Input: part model. Units: mm. Frame: model coordinates. Face numbers are marked on the shaded views. A direction names the side the tool comes from. Give positions to 0.01 mm unless a question says otherwise; leave off trailing zeros. Loops run counter-clockwise (first coordinate to the right, second up) from the corner with the lowest first, then second, coordinate; pieces in that order, holes last. Notation, with made-up numbers: M 87.5,-30.75 L 101.5,-30.75 A36 ccw 101.5,8.25 Z; hole C 56.5,61 d5. An arc over 180 degrees is marked long. One line per item, written item: value. Start each with the question number.
(1) Access query for the marked faces 1, 2 and 3. Directions: +Z, -Z, +X, -X, +Y, -Y. A direction counts if a zero-diameter tool reaches every point of the face in a straight line with its end or side. Return the directions, or none.
(2) Section B-B on z = -0.05. Output: boundary loops of the cut face in (x, y).
(3) Ray query, line 1 along Y through (x, z) = (0, 0.9); line 2 along Y through (x, z) = (0, -1.2); line 3 along Y through (x, z) = (-15.8, 0.7). Return the intervals inside material, ascending. Write a range as from..to.
(4) Pin query (flat end, axial travel): P1, Ø1.8, axis at x = 1, y = 15, coming from the +Z side; P2, Ø1.5, axis at y = 5.5, z = 1, coming from the -X side; P3, Ø3, axis at x = -15.8, y = 0, coming from the +Z side; P4, Ø1.4, axis at x = -15.5, z = -1, coming from the -Y side. Return the tip coordinate at first contact, or that it passes through.
(5) Section A-A on x = -15.8. Output: boundary loops of the cut face in (y, z).
(6) Pull-direction query (Y, two-part tool) for the marked faces 4, 5 and 6; classes: released by +Y, released by -Y, zero draft, split by the parting line, or undercut.
(7) Section D-D on y = 0. State how many separate pieces and enclosed holes the cut face has, plus the area to 3 significant figures.
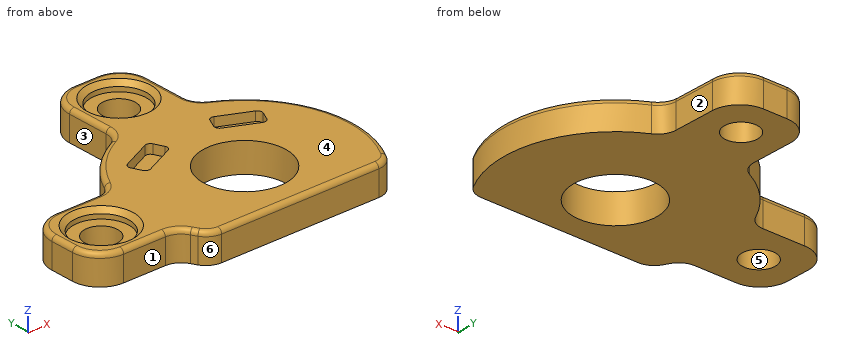
```python
from build123d import *

# Parameters (mm, degrees)
SKETCH10_R          = 4.5
BOSS_EXTRUDE6_DEPTH = 1.6
SKETCH13_R          = 1.8
BOSS_EXTRUDE7_DEPTH = 1.6
FILLET1_R           = 2
CUT_EXTRUDE2_DEPTH  = 1
SKETCH16_R          = 3
CUT_EXTRUDE3_DEPTH  = 1
CHAMFER1_SIZE       = 0.5
FILLET2_R           = 0.5


with BuildPart() as part:
    # Sketch10 → Boss-Extrude6 (new body, symmetric)
    with BuildSketch(Plane.XY):
        with BuildLine():
            Line((-9.746794345, -7), (9.746794345, -7))
            ThreePointArc((9.746794345, -7), (0, 12), (-9.746794345, -7))
        make_face()
        Circle(SKETCH10_R, mode=Mode.SUBTRACT)
    extrude(amount=BOSS_EXTRUDE6_DEPTH, both=True)

    # Sketch13 → Boss-Extrude7 (add, symmetric)
    with BuildSketch(Plane.XY):
        with BuildLine():
            Line((-11.203124564, 4.3), (-17.1, 4.3))
            ThreePointArc((-17.1, 4.3), (-19.221320344, 3.421320344), (-20.1, 1.3))
            Line((-20.1, 1.3), (-20.1, -1.3))
            ThreePointArc((-20.1, -1.3), (-19.221320344, -3.421320344), (-17.1, -4.3))
            Line((-17.1, -4.3), (-11.203124564, -4.3))
            ThreePointArc((-11.203124564, -4.3), (-12, 0), (-11.203124564, 4.3))
        make_face()
        with Locations((-15.8, 0)):
            Circle(SKETCH13_R, mode=Mode.SUBTRACT)
        with BuildLine():
            Line((4.3, 11.203124564), (4.3, 17.1))
            ThreePointArc((4.3, 17.1), (3.421320344, 19.221320344), (1.3, 20.1))
            Line((1.3, 20.1), (-1.3, 20.1))
            ThreePointArc((-1.3, 20.1), (-3.421320344, 19.221320344), (-4.3, 17.1))
            Line((-4.3, 17.1), (-4.3, 11.203124564))
            ThreePointArc((-4.3, 11.203124564), (0, 12), (4.3, 11.203124564))
        make_face()
        with Locations((0, 15.8)):
            Circle(SKETCH13_R, mode=Mode.SUBTRACT)
    extrude(amount=BOSS_EXTRUDE7_DEPTH, both=True)

    # Fillet1
    fillet1_edges = [part.edges().sort_by_distance(p)[0] for p in [
        (-11.203124564, -4.3, 0),
        (-11.203124564, 4.3, 0),
        (-4.3, 11.203124564, 0),
        (4.3, 11.203124564, 0),
        (9.746794345, -7, 0),
        (-9.746794345, -7, 0),
    ]]
    fillet(fillet1_edges, radius=FILLET1_R)

    # Sketch15 → Cut-Extrude2 (cut)
    with BuildSketch(Plane(origin=(0, 0, 1.6), x_dir=(-1, 0, 0), z_dir=(0, 0, -1))):
        with BuildLine():
            Line((-3.808047036, 8.187368684), (-7.070755069, 6.665942941))
            ThreePointArc((-7.070755069, 6.665942941), (-7.329292249, 6.38379912), (-7.312599832, 6.001479917))
            Line((-7.312599832, 6.001479917), (-6.847719744, 5.004541351))
            ThreePointArc((-6.847719744, 5.004541351), (-6.565575922, 4.746004172), (-6.18325672, 4.762696589))
            Line((-6.18325672, 4.762696589), (-2.920548686, 6.284122331))
            ThreePointArc((-2.920548686, 6.284122331), (-2.662011507, 6.566266153), (-2.678703924, 6.948585355))
            Line((-2.678703924, 6.948585355), (-3.143584012, 7.945523921))
            ThreePointArc((-3.143584012, 7.945523921), (-3.425727833, 8.204061101), (-3.808047036, 8.187368684))
        make_face()
        with BuildLine():
            Line((6.847719744, 5.004541351), (7.312599832, 6.001479917))
            ThreePointArc((7.312599832, 6.001479917), (7.329292249, 6.38379912), (7.070755069, 6.665942941))
            Line((7.070755069, 6.665942941), (3.808047036, 8.187368684))
            ThreePointArc((3.808047036, 8.187368684), (3.425727833, 8.204061101), (3.143584012, 7.945523921))
            Line((3.143584012, 7.945523921), (2.678703924, 6.948585355))
            ThreePointArc((2.678703924, 6.948585355), (2.662011507, 6.566266153), (2.920548686, 6.284122331))
            Line((2.920548686, 6.284122331), (6.18325672, 4.762696589))
            ThreePointArc((6.18325672, 4.762696589), (6.565575922, 4.746004172), (6.847719744, 5.004541351))
        make_face()
    extrude(amount=CUT_EXTRUDE2_DEPTH, mode=Mode.SUBTRACT)

    # Sketch16 → Cut-Extrude3 (cut)
    with BuildSketch(Plane(origin=(0, 0, 1.6), x_dir=(-1, 0, 0), z_dir=(0, 0, -1))):
        with Locations((0, 15.8)):
            Circle(SKETCH16_R)
        with Locations((15.8, 0)):
            Circle(SKETCH16_R)
    extrude(amount=CUT_EXTRUDE3_DEPTH, mode=Mode.SUBTRACT)

    # Chamfer1
    chamfer1_edges = [part.edges().sort_by_distance(p)[0] for p in [
        (3, 15.8, 1.6),
        (-12.8, 0, 1.6),
    ]]
    chamfer(chamfer1_edges, length=CHAMFER1_SIZE)

    # Fillet2
    fillet2_edges = [part.edges().sort_by_distance(p)[0] for p in [
        (-19.221320344, 3.421320344, 1.6),
        (-20.1, 0, 1.6),
        (-19.221320344, -3.421320344, 1.6),
        (-14.801199885, -4.3, 1.6),
        (3.421320344, 19.221320344, 1.6),
        (0, 20.1, 1.6),
        (-3.421320344, 19.221320344, 1.6),
        (-4.3, 14.801199885, 1.6),
        (-14.801199885, 4.3, 1.6),
        (-8.485281374, 8.485281374, 1.6),
        (4.3, 14.801199885, 1.6),
        (11.498184685, 3.433911609, 1.6),
        (-10.558586547, -5.702302178, 1.6),
        (0, -7, 1.6),
        (-9.660254038, -6.732050808, 1.6),
        (9.660254038, -6.732050808, 1.6),
        (-11.453590921, 4.597061363, 1.6),
        (4.597061363, 11.453590921, 1.6),
        (-4.597061363, 11.453590921, 1.6),
        (-11.453590921, -4.597061363, 1.6),
    ]]
    fillet(fillet2_edges, radius=FILLET2_R)


solid = part.part
```
Output values:
1. face 1: +Z, -Z, -X, -Y
1. face 2: +Z, -Z, +X, +Y
1. face 3: +Z, -Z, -X, +Y
2. outline: M -20.1,-1.3 A3 ccw -17.1,-4.3 L -12.5,-4.3 A2 cw -10.72,-5.4 A12 ccw -10.39,-6 A2 ccw -8.66,-7 L 8.66,-7 A2 ccw 10.39,-6 A12 ccw 5.4,10.72 A2 cw 4.3,12.5 L 4.3,17.1 A3 ccw 1.3,20.1 L -1.3,20.1 A3 ccw -4.3,17.1 L -4.3,12.5 A2 cw -5.4,10.72 A12 ccw -10.72,5.4 A2 cw -12.5,4.3 L -17.1,4.3 A3 ccw -20.1,1.3 Z; hole C -15.8,0 d3.6; hole C 0,0 d9; hole C 0,15.8 d3.6
3. line 1: y = -7..-4.5, 4.5..12.8, 18.8..20.1
3. line 2: y = -7..-4.5, 4.5..14, 17.6..20.1
3. line 3: y = -4.3..-3, 3..4.3
4. P1: stops at z = 0.6
4. P2: stops at x = -11.24
4. P3: passes through
4. P4: stops at y = -4.3
5. outline: M -4.3,-1.6 L -1.8,-1.6 L -1.8,0.6 L -3,0.6 L -3,1.1 L -3.5,1.6 L -3.8,1.6 A0.5 ccw -4.3,1.1 Z; M 1.8,-1.6 L 4.3,-1.6 L 4.3,1.1 A0.5 ccw 3.8,1.6 L 3.5,1.6 L 3,1.1 L 3,0.6 L 1.8,0.6 Z
6. face 4: zero draft
6. face 5: undercut
6. face 6: released by -Y
7. separate pieces: 3
7. enclosed holes: 0
7. area: 59.6 mm²
